The listing builds one solid part. Answer for the finished solid, in the listing's coordinates (mm). A direction names the side the tool comes from. Coordinates: 2 decimals unless noted, no trailing zeros. Order: outer loops, then holes, each group sorted by start corner. A loop starts at its lowest first (then second) coordinate and runs counter-clockwise, first axis right, second up. Notation, with made-up numbers: (51, -31) -> (90, -31) arc R23 cw to (90, -15) -> close; hole circle Ø10 at (-6.5, 3). An arc over 180 degrees is marked (long way). Return JSON: item names as keys, results as strings.
Autodesk Inventor part; units mm, degrees
ref_plane "YZ Plane" through (0, 0, 0) normal (1, 0, 0) x (0, 1, 0)
ref_plane "XZ Plane" through (0, 0, 0) normal (0, 1, 0) x (-1, 0, 0)
ref_plane "XY Plane" through (0, 0, 0) normal (0, 0, 1) x (1, 0, 0)
sketch "Sketch1" plane through (0, 0, 0) normal (0, 1, 0) x (-1, 0, 0)
  line L0 (-12.7, -12.7) -> (12.7, -12.7)
  line L1 (12.7, -12.7) -> (12.7, 12.7)
  line L2 (12.7, 12.7) -> (-12.7, 12.7)
  line L3 (-12.7, 12.7) -> (-12.7, -12.7)
  line L4 (-12.7, -12.7) -> (12.7, 12.7) construction
  line L5 (12.7, -12.7) -> (-12.7, 12.7) construction
  line L6 (9.525, 9.525) -> (9.525, -9.525)
  line L7 (9.525, -9.525) -> (-9.525, -9.525)
  line L8 (-9.525, -9.525) -> (-9.525, 9.525)
  line L9 (-9.525, 9.525) -> (9.525, 9.525)
  point P0 (0, 0)
  dimension "d0" = 25.4
  dimension "d1" = 25.4
  dimension "d2" = 3.175
extrude "Extrusion1" add sketch "Sketch1" along normal blind 514.35
sketch "Sketch2" plane through (-12.7, 0, 12.7) normal (0, 0, 1) x (1, 0, 0)
  line L0 (25.4, 488.95) -> (0, 488.95) construction
  line L1 (0, 488.95) -> (0, 514.35) construction
  line L2 (0, 514.35) -> (25.4, 514.35) construction
  line L3 (25.4, 514.35) -> (25.4, 488.95) construction
  line L4 (25.4, 488.95) -> (0, 514.35) construction
  line L5 (0, 488.95) -> (25.4, 514.35) construction
  circle A0 centre (12.7, 501.65) radius 2.4892
  circle A1 centre (12.7, 479.425) radius 3.2512
  circle A2 centre (12.7, 457.2) radius 3.2512
  point P0 (12.7, 0)
  dimension "d5" = 25.4
  dimension "d6" = 25.4
  dimension "d7" = 4.9784
  dimension "d10" = 22.225
  dimension "d11" = 22.225
  dimension "d12" = 6.5024
extrude "Extrusion2" cut sketch "Sketch2" against normal through all
properties part number "STRU_012_BilletPoleMiddle_Unique" material "Aluminum 6061"
Item 1: Find the intervals of material crossed by probe 1 along Y at (x, z) = (0, -10.5); probe 2 along X at (y, z) = (171.5, -3.5) (3 decimals), in increasing order.
Answer list:
{"probe 1": "0 to 453.95, 460.45 to 476.17, 482.68 to 499.16, 504.14 to 514.35", "probe 2": "-12.7 to -9.525, 9.525 to 12.7"}
Item 2: Which of the six approach directions +Z, -Z, +X, -X, +Y, -Y give full straight-line access (tool end or side, diameter ignored) to faces 1 (the flat face through (0, 254, 12.7)), 2 (the flat face through (-9.525, 254, 0))?
Answer list:
{"face 1": "+Z, +X, -X, +Y, -Y", "face 2": "+Y, -Y"}
Item 3: The part is cut by section A-A on z = -1.25. Determine the outline of the cut face in (x, y) (3 decimals).
Answer list:
{"outline": "(-12.7, 0) -> (-9.525, 0) -> (-9.525, 514.35) -> (-12.7, 514.35) -> close; (9.525, 0) -> (12.7, 0) -> (12.7, 514.35) -> (9.525, 514.35) -> close"}
Item 4: The part is cut by section B-B on y = 228. Determine the outline of the cut face in (x, z) (3 decimals), plus the area to 3 significant figures.
Answer list:
{"outline": "(-12.7, -12.7) -> (12.7, -12.7) -> (12.7, 12.7) -> (-12.7, 12.7) -> close; hole (-9.525, -9.525) -> (9.525, -9.525) -> (9.525, 9.525) -> (-9.525, 9.525) -> close", "area": "282 mm2"}
Item 5: Determine the mould class of faces 3 (the flat face through (-12.7, 254, 0)), 4 (the flat face through (0, 254, -9.525)), 5 (the flat face through (-11, 0, 0)) for opening direction X: pulls with the +X half, pulls with the -X half, needs draft (parallel to the pull), parting line crosses it, or undercut.
Answer list:
{"face 3": "pulls with the -X half", "face 4": "undercut", "face 5": "needs draft"}
